```python
from build123d import *

# Parameters (mm, degrees)
SKETCH1_W           = 250
SKETCH1_H           = 60
BOSS_EXTRUDE1_DEPTH = 4
SKETCH3_R           = 3.51887986
CUT_EXTRUDE1_DEPTH  = 10
SKETCH4_W           = 10
SKETCH4_H           = 11.7
CUT_EXTRUDE2_DEPTH  = 10
SKETCH5_W           = 7
SKETCH5_H           = 7
CUT_EXTRUDE3_DEPTH  = 10
CUT_EXTRUDE4_DEPTH  = 10


with BuildPart() as part:
    # Sketch1 → Boss-Extrude1 (new body)
    with BuildSketch(Plane.XY):
        with Locations((12.569832402, 50.449192367)):
            Rectangle(SKETCH1_W, SKETCH1_H)
    extrude(amount=BOSS_EXTRUDE1_DEPTH)

    # Sketch3 → Cut-Extrude1 (cut)
    with BuildSketch(Plane.XY.offset(4)):
        with Locations((-89.798295426, 40.153008957)):
            Circle(SKETCH3_R)
        with Locations((-117.322145335, -107.100984963)):
            Circle(SKETCH3_R)
        with Locations((-60.625269482, 39.492893663)):
            Circle(SKETCH3_R)
    extrude(amount=-CUT_EXTRUDE1_DEPTH, mode=Mode.SUBTRACT)

    # Sketch4 → Cut-Extrude2 (cut)
    with BuildSketch(Plane.XY.offset(4)):
        with Locations((-3.832712542, 40.15230201)):
            Rectangle(SKETCH4_W, SKETCH4_H)
        with Locations((-26.944599832, 40.15230201)):
            Rectangle(SKETCH4_W, SKETCH4_H)
        with Locations((37.914072819, 40.15230201)):
            Rectangle(SKETCH4_W, SKETCH4_H)
        with Locations((18.306555148, 40.15230201)):
            Rectangle(SKETCH4_W, SKETCH4_H)
    extrude(amount=-CUT_EXTRUDE2_DEPTH, mode=Mode.SUBTRACT)

    # Sketch5 → Cut-Extrude3 (cut)
    with BuildSketch(Plane.XY.offset(4)):
        with Locations((100.58753259, 39.945504984)):
            Rectangle(SKETCH5_W, SKETCH5_H)
    extrude(amount=-CUT_EXTRUDE3_DEPTH, mode=Mode.SUBTRACT)

    # Sketch6 → Cut-Extrude4 (cut)
    with BuildSketch(Plane.XY.offset(4)):
        Polygon((118.560482945, 33.81903225), (117.525576266, 35.420059377), (114.174927615, 35.251571832), (112.645517783, 32.265581209), (114.466756603, 29.44807813), (117.817405254, 29.616565675), (118.634511019, 31.211867406), (117.848178879, 32.428343358), align=None)
        Polygon((119.42955977, 35.515801288), (118.560482945, 33.81903225), (119.346815086, 32.602556298), (118.634511019, 31.211867406), (119.731305434, 29.515098368), (123.19581288, 29.689311308), (124.777193772, 32.776769239), (122.894067216, 35.690014229), align=None)
        Polygon((119.346815086, 32.602556298), (118.560482945, 33.81903225), (117.848178879, 32.428343358), (118.634511019, 31.211867406), align=None)
    extrude(amount=-CUT_EXTRUDE4_DEPTH, mode=Mode.SUBTRACT)


solid = part.part
```
Geometry check sheet. Reference: the model listing, model coordinates, mm. A direction names the side the tool comes from. Coordinates: 2 decimals unless noted, no trailing zeros. Order: outer loops, then holes, each group sorted by start corner. A loop starts at its lowest first (then second) coordinate and runs counter-clockwise, first axis right, second up. Notation, with made-up numbers: (-10, -23) - (11, -23) arc R23 cw to (11, -2) - close; hole circle Ø2 at (10.5, -27). An arc over 180 degrees is marked (long way). Use one line per item in the form item = value.
1. Section check A-A (x = 21). Record the boundary of the cut face in (y, z), then the cut area to 3 significant figures.
Here are the results:
outline = (20.45, 0) - (34.3, 0) - (34.3, 4) - (20.45, 4) - close; (46, 0) - (80.45, 0) - (80.45, 4) - (46, 4) - close
area = 193 mm²
2. Draft check along X on faces 3 (the face through (11, 80.449, 2)), 4 (the face through (13.307, 40, 2)), 5 (the face through (-112.43, 50, 2)). Enter one of: pulls with the +X half, pulls with the -X half, needs draft (parallel to the pull), parting line crosses it, or undercut.
Here are the results:
face_3 = needs draft
face_4 = undercut
face_5 = pulls with the -X half
3. Access from +Z, -Z, +X, -X, +Y, -Y to the whole of each face (thin tool, end or side, straight path). Record for faces 1 (the face through (11, 51, 0)), 2 (the face through (23.307, 40, 2)).
Here are the results:
face_1 = -Z, +X, -X, +Y, -Y
face_2 = +Z, -Z
4. Scan lines: line 1 (Y direction, x = 122, z = 3.4); line 2 (Y direction, x = 36, z = 2.4); line 3 (X direction, y = 32, z = 2.05). Record each from-to range of solid material in increasing order.
Here are the results:
line_1 = 20.45 to 29.63, 35.65 to 80.45
line_2 = 20.45 to 34.3, 46 to 80.45
line_3 = -112.43 to 112.82, 124.38 to 137.57
5. Section check B-B (z = 1.95). State how many separate pieces and enclosed holes the cut face has, then the cut area to 3 significant figures.
Here are the results:
separate_pieces = 1
enclosed_holes = 8
area = 14,300 mm²
